```python
from build123d import *

# Parameters (mm, degrees)
ESQUISSE1_R          = 2.6
BASE_EXTRUSION_DEPTH = 3


with BuildPart() as part:
    # Esquisse1 → Base-Extrusion (new body)
    with BuildSketch(Plane.XY):
        with BuildLine():
            Line((42.260472267, 1.47721163), (38.305407289, 2.174596295))
            ThreePointArc((38.305407289, 2.174596295), (36.604258385, 2.910637942), (35.417544816, 4.334497417))
            ThreePointArc((35.417544816, 4.334497417), (34.703252614, 5.26032071), (33.689272741, 5.842735456))
            ThreePointArc((33.689272741, 5.842735456), (22.679517475, 8.332820348), (11.393281032, 8.522822221))
            ThreePointArc((11.393281032, 8.522822221), (10.314139297, 8.856754257), (9.773978095, 9.848864818))
            Line((9.773978095, 9.848864818), (9.402019506, 13.140725264))
            ThreePointArc((9.402019506, 13.140725264), (9.043446847, 13.565088236), (8.514166767, 13.396206973))
            Line((8.514166767, 13.396206973), (3.974497387, 7.699944601))
            ThreePointArc((3.974497387, 7.699944601), (3.608247601, 7.370259002), (3.154924555, 7.177050008))
            ThreePointArc((3.154924555, 7.177050008), (0.572430777, 6.483979152), (-1.973326778, 5.666214029))
            ThreePointArc((-1.973326778, 5.666214029), (-5.560323829, -2.254506357), (2.530032468, -5.440490393))
            ThreePointArc((2.530032468, -5.440490393), (21.756803647, -0.153586273), (41.654398955, -1.459643764))
            ThreePointArc((41.654398955, -1.459643764), (43.469044461, -0.303163936), (42.260472267, 1.47721163))
        make_face()
        Circle(ESQUISSE1_R, mode=Mode.SUBTRACT)
    extrude(amount=BASE_EXTRUSION_DEPTH)


solid = part.part
```
For this review, take the finished solid that the model builds, in its own axes (mm). A direction names the side the tool comes from. Coordinates: 2 decimals unless noted, no trailing zeros. Write each loop counter-clockwise with the first axis right and the second up, starting at its lowest first coordinate (ties: lowest second). Pieces come first, ordered by that corner, then holes.
(1) Add section A-A on z = 2.55. Give the boundary of the cut face in (x, y).
(2) Tool access review of faces 1 (the face through (10.327, 8.847, 1.479)), 2 (the face through (40.31, 1.82, 1.48)): name each direction out of +Z, -Z, +X, -X, +Y, -Y from which nothing blocks a thin tool from reaching the whole face with its end or side.
(3) Wall thickness on probe 1 along Y at (x, z) = (0, 2.05); probe 2 along Y at (x, z) = (1.5, 1.9); probe 3 along Y at (x, z) = (28, 0.75): over which ranges is each line inside the solid? List them lowest first.
(4) Add section B-B on x = 0. Give the boundary of the cut face in (y, z), then the cut area to 3 significant figures.
(5) The part is to be moulded in two halves that separate along X. For faces 3 (the face through (13, 2, 3)), 4 (the face through (34.716, 5.249, 1.479)), 5 (the face through (22.837, 8.314, 1.479)), say which applies: +X half, -X half, draft (parallel to the pull), parting line (faces both ways), or undercut.
(6) Add section C-C on y = 12.5. Give the boundary of the cut face in (x, z).
(7) For pin 1 Ø5 at (x, y) = (26, 4.5) entering from -Z, flat-tipped, find the tip position at first contact; note if it passes through.
(8) Add section D-D on x = 22. Give the boundary of the cut face in (y, z), then the cut area to 3 significant figures.
Answer sheet:
1. outline: (-1.97, 5.67) arc R6 ccw (long way) to (2.53, -5.44) arc R60 cw to (41.65, -1.46) arc R1.5 ccw (long way) to (42.26, 1.48) - (38.31, 2.17) arc R4 cw to (35.42, 4.33) arc R3 ccw to (33.69, 5.84) arc R55 ccw to (11.39, 8.52) arc R1.5 cw to (9.77, 9.85) - (9.4, 13.14) arc R0.5 ccw to (8.51, 13.4) - (3.97, 7.7) arc R1.5 cw to (3.15, 7.18) arc R55 ccw to start; hole circle Ø5.2 at (0, 0)
2. face 1: +Z, -Z, +Y
2. face 2: +Z, -Z, +X, +Y
3. probe 1: y = -6 to -2.6, 2.6 to 6.31
3. probe 2: y = -5.81 to -2.12, 2.12 to 6.75
3. probe 3: y = 0.15 to 7.43
4. outline: (-6, 0) - (-2.6, 0) - (-2.6, 3) - (-6, 3) - close; (2.6, 0) - (6.31, 0) - (6.31, 3) - (2.6, 3) - close
4. area: 21.3 mm2
5. face 3: draft
5. face 4: +X half
5. face 5: undercut
6. outline: (7.8, 0) - (9.47, 0) - (9.47, 3) - (7.8, 3) - close
7. pin 1: stops at z = 0
8. outline: (-0.13, 0) - (8.41, 0) - (8.41, 3) - (-0.13, 3) - close
8. area: 25.6 mm2
